from build123d import *

# Parameters (mm, degrees)
F1_DEPTH  = 16
F2_W      = 70
F2_H      = 3
F3_DEPTH  = 2
F4_W      = 50
F4_H      = 14
F5_DEPTH  = 2
F6_R      = 1
F9_DEPTH  = 2
F11_DEPTH = 38.001
F13_D     = 4
F14_R     = 3
F14_R_2   = 2
F15_DEPTH = 5
F16_R     = 3


# Not quite as in the source:
# - a pattern or mirror of a feature is missing from the dataset's text; its kind, count and spacing are read off the source's solid


with BuildPart() as f1:
    # F0 (on Front) → F1 (new body)
    with BuildSketch(Plane.XZ):
        with BuildLine():
            Line((94, 9), (0, 9))
            ThreePointArc((0, 9), (-9, 0), (0, -9))
            Line((0, -9), (19, -9))
            ThreePointArc((19, -9), (20.7502012229, -9.5634459417), (21.8429732618, -11.0421362138))
            ThreePointArc((21.8429732618, -11.0421362138), (47.7390385011, -46.2740019539), (89.2552166837, -59.996155849))
            ThreePointArc((89.2552166837, -59.996155849), (94.7998907394, -61.2192390349), (99.4028141151, -64.5437599417))
            Line((99.4028141151, -64.5437599417), (100.6981825128, -63))
            ThreePointArc((100.6981825128, -63), (95.5856099225, -59.3797463332), (89.4748869571, -58))
            ThreePointArc((89.4748869571, -58), (48.7477072094, -44.5420257674), (23.5164318764, -9.8548093079))
            ThreePointArc((23.5164318764, -9.8548093079), (21.6715207784, -7.7735385095), (19, -7))
            Line((19, -7), (0, -7))
            ThreePointArc((0, -7), (-7, 0), (0, 7))
            Line((0, 7), (94, 7))
            Line((94, 7), (94, 9))
        make_face()
    extrude(amount=F1_DEPTH)

    # F2 (on face) → F3 (join)
    with BuildSketch(Plane.XY.offset(9)):
        with Locations((59, -17.5)):
            Rectangle(F2_W, F2_H)
    extrude(amount=-F3_DEPTH)

    # F4 (on face) → F5 (join)
    with BuildSketch(Plane.XZ.offset(19)):
        with Locations((69, 2)):
            Rectangle(F4_W, F4_H)
    extrude(amount=-F5_DEPTH)

    # F6
    f6_edges = [f1.edges().sort_by_distance(p)[0] for p in [
        (69, -17, 7),
    ]]
    fillet(f6_edges, radius=F6_R)

    # F7: F1 across plane


with BuildPart() as f1_1:
    add(f1.part)
    add(f1.part.mirror(Plane.XZ))

    # F8 (on face) → F9 (cut)
    with BuildSketch(Plane.XY.offset(9)):
        with BuildLine():
            Line((94, 12), (34, 12))
            ThreePointArc((34, 12), (22, 0), (34, -12))
            Line((34, -12), (94, -12))
            Line((94, -12), (94, 12))
        make_face()
    extrude(amount=-F9_DEPTH, mode=Mode.SUBTRACT)

    # F10 (on face) → F11 (cut, through all)
    with BuildSketch(Plane.XZ.offset(19)):
        with BuildLine():
            ThreePointArc((50, 3), (47, 0), (50, -3))
            Line((50, -3), (70, -3))
            ThreePointArc((70, -3), (73, 0), (70, 3))
            Line((70, 3), (50, 3))
        make_face()
    extrude(amount=-F11_DEPTH, mode=Mode.SUBTRACT)

    # F13 (through all)
    with Locations(Plane.XZ.offset(19)):
        with Locations((80, 1)):
            Hole(F13_D / 2)

    # F14 (on face) → F15 (join)
    with BuildSketch(Plane(origin=(0, -17, 0), x_dir=(-1, 0, 0), z_dir=(0, 1, 0))):
        with Locations((-80, 1)):
            Circle(F14_R)
        with Locations((-80, 1)):
            Circle(F14_R_2, mode=Mode.SUBTRACT)
    f15 = extrude(amount=F15_DEPTH)

    # F15_copies: F15 across plane
    add(f15.mirror(Plane.ZX))

    # F16
    f16_edges = [f1_1.edges().sort_by_distance(p)[0] for p in [
        (94, -18, -5),
        (44, -18, -5),
        (94, 18, -5),
        (44, 18, -5),
    ]]
    fillet(f16_edges, radius=F16_R)


solid = f1_1.part
Verification items for the finished model (mm, model axes). A direction names the side the tool comes from. Coordinates: 2 decimals unless noted, no trailing zeros. Order: outer loops, then holes, each group sorted by start corner. A loop starts at its lowest first (then second) coordinate and runs counter-clockwise, first axis right, second up. Notation, with made-up numbers: M 2.25,5.25 L 23.25,5.25 A19 cw 23.25,18.25 Z; hole C 80,1 d4. An arc over 180 degrees is marked long. One line per item, written item: value. Start each with the question number.
Item 1: Scan lines: probe 1 along Z at (x, y) = (9.5, 6); probe 2 along Z at (x, y) = (80, -13.3); probe 3 along Z at (x, y) = (80, -18). Record each from-to range of solid material in increasing order.
Item 2: Sectioned sample at C-C (x = 25.5). Enter the section's corners in (y, z), then the cut area to 3 significant figures.
Item 3: Sectioned sample at A-A (x = 6). Enter the section's corners in (y, z).
Item 4: Access from +Z, -Z, +X, -X, +Y, -Y to the whole of each face (thin tool, end or side, straight path). Record for faces 4 (the flat face through (9, 0, -9)), 5 (the flat face through (29, -16, -25)), 6 (the flat face through (79, -12, -1)), 7 (the flat face through (25, -9, 7)), 8 (the cylindrical face through (73, -18, 0)).
Item 5: Gauge pin test, flat ends, axial feed: pin 1 (0.6 mm diameter, centred on x = 60.5, y = 18, fed in from -Z); pin 2 (21 mm diameter, centred on x = 6, y = -5.5, fed in from -Z); pin 3 (3.5 mm diameter, centred on y = -18, z = 2, fed in from -X). Record the tip position at first contact, or that the pin passes through.
Item 6: Mould release check, pull along Z, two halves, no side actions. Record for faces 1 (the cylindrical face through (83, -15, 1)), 2 (the flat face through (44, -18, 2)), 3 (the cylindrical face through (47.24, -0.22, -45.91)): released by +Z, released by -Z, zero draft, split by the parting line, or undercut.
Item 7: Sectioned sample at D-D (x = 80). Count the separate pieces of the cut face and the enclosed holes in it, then the cut area to 3 significant figures.
Item 8: Sectioned sample at B-B (y = 0). Enter the section's corners in (x, z).
Conclusion:
1. probe 1: z = -9 to -7, 7 to 9
1. probe 2: z = -59.3 to -57.28, -2 to -1, 3 to 4, 7 to 9
1. probe 3: z = -5 to -1, 3 to 9
2. outline: M -19,7 L -8.47,7 L -8.47,9 L -19,9 Z; M -16,-19.9 L 16,-19.9 L 16,-15.16 L -16,-15.16 Z; M 8.47,7 L 19,7 L 19,9 L 8.47,9 Z
2. area: 194 mm^2
3. outline: M -16,-9 L 16,-9 L 16,-7 L -16,-7 Z; M -16,7 L 16,7 L 16,9 L -16,9 Z
4. face 4: -Z, -X, +Y, -Y
4. face 5: -Z, -X, -Y
4. face 6: +Z, +X
4. face 7: none
4. face 8: +Y, -Y
5. pin 1: stops at z = -5
5. pin 2: stops at z = -9
5. pin 3: stops at x = 44
6. face 1: undercut
6. face 2: zero draft
6. face 3: released by -Z
7. separate pieces: 5
7. enclosed holes: 0
7. area: 145 mm^2
8. outline: M 0,-9 L 19,-9 A3 cw 21.84,-11.04 A71.92 ccw 89.26,-60 A14 cw 99.4,-64.54 L 100.7,-63 A16 ccw 89.47,-58 A70 cw 23.52,-9.85 A5 ccw 19,-7 L 0,-7 A7 cw 0,7 L 22,7 L 22,9 L 0,9 A9 ccw Z
